```python
from build123d import *

# Parameters (mm, degrees)
BOSS_EXTRUDE1_DEPTH = 4


with BuildPart() as part:
    # Sketch1 → Boss-Extrude1 (new body)
    with BuildSketch(Plane.XY):
        Polygon((0, 0), (8, 0), (8, 4), (11, 4), (11, 8), (8, 8), (8, 12), (0, 12), (0, 8), (-3, 8), (-3, 4), (0, 4), align=None)
        Polygon((7, 6), (5.5, 8.598076211), (2.5, 8.598076211), (1, 6), (2.5, 3.401923789), (5.5, 3.401923789), align=None, mode=Mode.SUBTRACT)
    extrude(amount=BOSS_EXTRUDE1_DEPTH)


solid = part.part
```
Can you work these out from the model? Positions are in its coordinate system, mm. A direction names the side the tool comes from. Coordinates: 2 decimals unless noted, no trailing zeros. Loops run counter-clockwise (first coordinate to the right, second up) from the corner with the lowest first, then second, coordinate; pieces in that order, holes last.
1) Thinking about a two-plate mould opening in X: for faces 5 (the flat face through (6.24, 4.68, 1.97)), 6 (the flat face through (9, 4, 2)), 7 (the flat face through (-3, 6, 2)), which applies, pulls with the +X half, pulls with the -X half, needs draft (parallel to the pull), parting line crosses it, or undercut?
2) Imagine slicing it at D-D on y = 9.75. List the corners of the cut face in (x, z) for me.
3) Which directions (+Z, -Z, +X, -X, +Y, -Y) give clear straight access to the entire face, cutting with the end or side of a thin tool? Please do faces 1 (the flat face through (8, 10, 2)), 2 (the flat face through (-2, 4, 2)), 3 (the flat face through (0, 10, 2)), 4 (the flat face through (4, 3.402, 2)).
4) For pin 1 (0.9 mm diameter, centred on x = 9.5, z = 2.5, fed in from -Y); pin 2 (2 mm diameter, centred on x = -1, y = 7, fed in from -Z); pin 3 (2 mm diameter, centred on y = 10.5, z = 3, fed in from +X); pin 4 (1.2 mm diameter, centred on y = 9, z = 2, fed in from -X), each with a flat end and sliding along its axis, tell me the tip position at first contact or that it passes through.
5) I need wall thicknesses on probe 1 along Y at (x, z) = (4, 0.8); probe 2 along X at (y, z) = (2.75, 3.8); probe 3 along Y at (x, z) = (-0.5, 2.8). Which ranges of each line are inside material? Lowest first, please.
6) Imagine slicing it at B-B on z = 0.3. List the corners of the cut face in (x, y) for me.
7) Imagine slicing it at A-A on x = 5. List the corners of the cut face in (y, z) for me.
8) Imagine slicing it at C-C on y = 5.25. List the corners of the cut face in (x, z) for me.
Completed:
1. face 5: undercut
1. face 6: needs draft
1. face 7: pulls with the -X half
2. outline: (0, 0) - (8, 0) - (8, 4) - (0, 4) - close
3. face 1: +Z, -Z, +X, +Y
3. face 2: +Z, -Z, -X, -Y
3. face 3: +Z, -Z, -X, +Y
3. face 4: +Z, -Z
4. pin 1: stops at y = 4
4. pin 2: stops at z = 0
4. pin 3: stops at x = 8
4. pin 4: stops at x = 0
5. probe 1: y = 0 to 3.4, 8.6 to 12
5. probe 2: x = 0 to 8
5. probe 3: y = 4 to 8
6. outline: (-3, 4) - (0, 4) - (0, 0) - (8, 0) - (8, 4) - (11, 4) - (11, 8) - (8, 8) - (8, 12) - (0, 12) - (0, 8) - (-3, 8) - close; hole (1, 6) - (2.5, 3.4) - (5.5, 3.4) - (7, 6) - (5.5, 8.6) - (2.5, 8.6) - close
7. outline: (0, 0) - (3.4, 0) - (3.4, 4) - (0, 4) - close; (8.6, 0) - (12, 0) - (12, 4) - (8.6, 4) - close
8. outline: (-3, 0) - (1.43, 0) - (1.43, 4) - (-3, 4) - close; (6.57, 0) - (11, 0) - (11, 4) - (6.57, 4) - close
